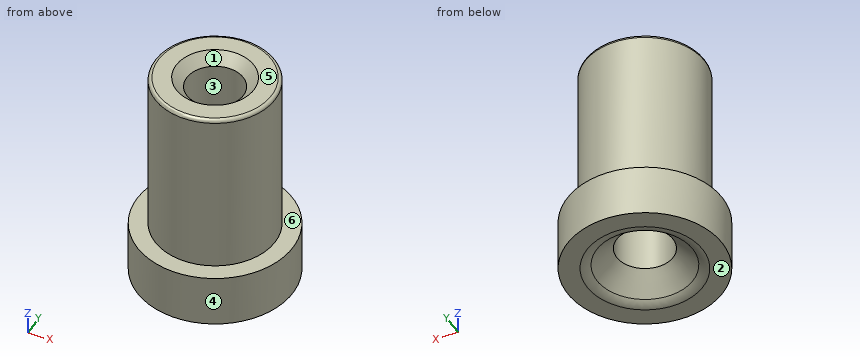
from build123d import *

# Parameters (mm, degrees)
F2_R = 0.25
F3_R = 1


with BuildPart() as f1:
    # F0 (on Front) → F1 (revolve)
    with BuildSketch(Plane.XZ):
        Polygon((-2, 8.25), (-2.75, 9), (-4.25, 9), (-4.25, 6.75), (-4.25, 6), (-4.25, -3), (-5.5, -3), (-5.5, -6.75), (-4.25, -6.75), (-3.706053, -6.75), (-2, -5.100015), align=None)
    revolve(axis=Axis((0, 0, 1.255823), (0, 0, -1)))

    # F2
    f2_edges = [f1.edges().sort_by_distance(p)[0] for p in [
        (4.25, 0, 9),
    ]]
    fillet(f2_edges, radius=F2_R)

    # F3
    f3_edges = [f1.edges().sort_by_distance(p)[0] for p in [
        (3.706053, 0, -6.75),
    ]]
    fillet(f3_edges, radius=F3_R)


solid = f1.part
Geometry: final body of the model. Coordinates: model frame, mm. Face numbers are marked on the shaded views. A direction names the side the tool comes from. Give positions to 0.01 mm unless a question says otherwise; leave off trailing zeros. Write each loop counter-clockwise with the first axis right and the second up, starting at its lowest first coordinate (ties: lowest second). Pieces come first, ordered by that corner, then holes.
(1) Cut plane C-C, the plane z = -4.5. Return loops of the section in (x, y), then the cut area to 3 significant figures.
(2) First-contact query: P1, Ø4, axis at x = 4.5, y = -2, coming from the +Z side; P2, Ø1.5, axis at x = 1.5, y = 1.5, coming from the -Z side; P3, Ø3, axis at x = 0, y = 0, coming from the -Z side; P4, Ø6, axis at y = 4.5, z = -5, coming from the -X side. Flat tips, straight axial feed; report the tip coordinate or a pass-through.
(3) Ray query, line 1 (Y direction, x = 0, z = 4.5); line 2 (Z direction, x = -5, y = -0.5); line 3 (Y direction, x = 0.75, z = 2). Return the intervals inside material, ascending.
(4) Cut plane A-A, the plane x = 0. Return loops of the section in (y, z), then the cut area to 3 significant figures.
(5) Cut plane D-D, the plane z = 4. Return loops of the section in (x, y), then the cut area to 3 significant figures.
(6) Access query for the marked faces 5 and 6. Directions: +Z, -Z, +X, -X, +Y, -Y. A direction counts if a zero-diameter tool reaches every point of the face in a straight line with its end or side. Return the directions, or none.
(7) Mould query, pull axis Y, two halves, no side actions, for the marked faces 1, 2, 3 and 4. Classes: released by +Y, released by -Y, zero draft, split by the parting line, or undercut.
Values follow:
1. outline: circle Ø11 at (0, 0); hole circle Ø4 at (0, 0)
1. area: 82.5 mm2
2. P1: stops at z = 9
2. P2: stops at z = -5.94
2. P3: passes through
2. P4: stops at x = -5.29
3. line 1: y = -4.25 to -2, 2 to 4.25
3. line 2: z = -6.75 to -3
3. line 3: y = -4.18 to -1.85, 1.85 to 4.18
4. outline: (-5.5, -6.75) - (-4.11, -6.75) arc R1 ccw to (-3.42, -6.47) - (-2, -5.1) - (-2, 8.25) - (-2.75, 9) - (-4, 9) arc R0.25 ccw to (-4.25, 8.75) - (-4.25, -3) - (-5.5, -3) - close; (2, -5.1) - (3.42, -6.47) arc R1 ccw to (4.11, -6.75) - (5.5, -6.75) - (5.5, -3) - (4.25, -3) - (4.25, 8.75) arc R0.25 ccw to (4, 9) - (2.75, 9) - (2, 8.25) - close
4. area: 76.8 mm2
5. outline: circle Ø8.5 at (0, 0); hole circle Ø4 at (0, 0)
5. area: 44.2 mm2
6. face 5: +Z, +X, -X, +Y, -Y
6. face 6: +Z
7. face 1: undercut
7. face 2: zero draft
7. face 3: undercut
7. face 4: split by the parting line
